For this review, take the finished solid that the model builds, in its own axes (mm). Face numbers are marked on the shaded views. A direction names the side the tool comes from. Round coordinates to 2 decimals unless told otherwise and drop trailing zeros. Loops run counter-clockwise (first coordinate to the right, second up) from the corner with the lowest first, then second, coordinate; pieces in that order, holes last.
1) Take a section at B-B (y = 28.2). State the section outline as (x, z) points.
2) Take a section at C-C (z = 23.5). State the section outline as (x, y) points, then the cut area to 3 significant figures.
3) Insertion check: pin 1 (4.5 mm diameter, centred on y = 51.7, z = 23.5, fed in from -X); pin 2 (4 mm diameter, centred on y = 53, z = -23.5, fed in from -X). Each pin has a flat end and moves straight along its axis. Give the tip position at first contact, or say it passes through.
4) Wall thickness on L1, parallel to Y at x = -43.5, z = 23.5; L2, parallel to Z at x = -50, y = 4; L3, parallel to Y at x = -42, z = 23: over which ranges is each line inside the solid? List them lowest first.
5) Take a section at A-A (x = -48). State the section outline as (y, z) points, then the cut area to 3 significant figures.
6) Take a section at D-D (z = 2). State the section outline as (x, y) points, then the cut area to 3 significant figures.
7) Tool access review of the marked faces 1 and 2: name each direction out of +Z, -Z, +X, -X, +Y, -Y from which nothing blocks a thin tool from reaching the whole face with its end or side.
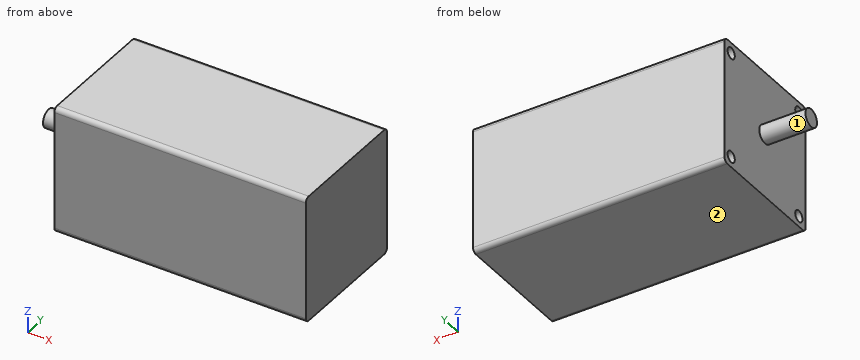
```python
from build123d import *

# Parameters (mm, degrees)
SKETCH1_W                    = 112
SKETCH1_H                    = 56.4
BOSS_EXTRUDE1_DEPTH          = 56.4
FILLET1_R                    = 2
SKETCH2_R                    = 4
BOSS_EXTRUDE2_DEPTH          = 20.6
F_5_0_5_DIAMETER_HOLE1_D     = 5
F_5_0_5_DIAMETER_HOLE1_DEPTH = 16


with BuildPart() as part:
    # Sketch1 → Boss-Extrude1 (new body)
    with BuildSketch(Plane(origin=(0, 0, 0), x_dir=(1, 0, 0), z_dir=(0, 1, 0))):
        Rectangle(SKETCH1_W, SKETCH1_H)
    extrude(amount=BOSS_EXTRUDE1_DEPTH)

    # Fillet1
    fillet1_edges = [part.edges().sort_by_distance(p)[0] for p in [
        (0, 56.4, 28.2),
        (0, 0, 28.2),
        (0, 0, -28.2),
        (0, 56.4, -28.2),
    ]]
    fillet(fillet1_edges, radius=FILLET1_R)

    # Sketch2 → Boss-Extrude2 (add)
    with BuildSketch(Plane.ZY.offset(56)):
        with Locations(Location((0, 28.2, 0), (0, 0, 180))):
            Circle(SKETCH2_R)
    extrude(amount=BOSS_EXTRUDE2_DEPTH)

    # 5.0 _5_ Diameter Hole1
    with Locations(Plane.ZY.offset(56)):
        with Locations((-23.5, 51.7), (23.5, 51.7), (23.501841312, 4.700000036), (-23.498158688, 4.700000036)):
            Hole(F_5_0_5_DIAMETER_HOLE1_D / 2, depth=F_5_0_5_DIAMETER_HOLE1_DEPTH)


solid = part.part
```
Response:
1. outline: (-76.6, -4) - (-56, -4) - (-56, -28.2) - (56, -28.2) - (56, 28.2) - (-56, 28.2) - (-56, 4) - (-76.6, 4) - close
2. outline: (-56, 0) - (56, 0) - (56, 56.4) - (-56, 56.4) - (-56, 54.2) - (-40, 54.2) - (-40, 49.2) - (-56, 49.2) - (-56, 7.2) - (-40, 7.2) - (-40, 2.2) - (-56, 2.2) - close
2. area: 6,160 mm2
3. pin 1: stops at x = -40
3. pin 2: stops at x = -56
4. L1: y = 0 to 2.2, 7.2 to 49.2, 54.2 to 56.4
4. L2: z = -28.2 to -25.9, -21.1 to 21.1, 25.9 to 28.2
4. L3: y = 0 to 2.25, 7.15 to 49.25, 54.15 to 56.4
5. outline: (0, -26.2) arc R2 ccw to (2, -28.2) - (54.4, -28.2) arc R2 ccw to (56.4, -26.2) - (56.4, 26.2) arc R2 ccw to (54.4, 28.2) - (2, 28.2) arc R2 ccw to (0, 26.2) - close; hole circle Ø5 at (4.7, -23.5); hole circle Ø5 at (4.7, 23.5); hole circle Ø5 at (51.7, -23.5); hole circle Ø5 at (51.7, 23.5)
5. area: 3,100 mm2
6. outline: (-76.6, 24.74) - (-56, 24.74) - (-56, 0) - (56, 0) - (56, 56.4) - (-56, 56.4) - (-56, 31.66) - (-76.6, 31.66) - close
6. area: 6,460 mm2
7. face 1: -X
7. face 2: -Z, +X, -X, +Y, -Y
